Work out the finished part from the listing and answer in its coordinate system (mm). Coordinates: 2 decimals unless noted, no trailing zeros. Order: outer loops, then holes, each group sorted by start corner. A loop starts at its lowest first (then second) coordinate and runs counter-clockwise, first axis right, second up. Notation, with made-up numbers: M 4.25,31 L 54.25,31 A17 ccw 54.25,64 Z; hole C 83,-32.5 d2. An arc over 180 degrees is marked long. Write item = value, one per line. Start each with the question number.
Q1. Find section C-C on y = 0.7. Give the vertices of the cut face in (x, z) (3 decimals).
Q2. Straight lines are drawn through the part: line 1 along Z through (x, y) = (67, 0.35) (3 decimals); line 2 along X through (y, z) = (1.7, 1) (3 decimals); line 3 along Z through (x, y) = (64.5, 0.95). For each, find the intervals that lie inside material, in ascending order.
Q3. Find section A-A on z = 0. Give the vertices of the cut face in (x, y) (3 decimals).
Q4. Find section B-B on x = 70.5. Give the vertices of the cut face in (y, z) (3 decimals).
Q5. Find section D-D on x = 82.5. Give the vertices of the cut face in (y, z) (3 decimals), and give its area (3 significant figures).
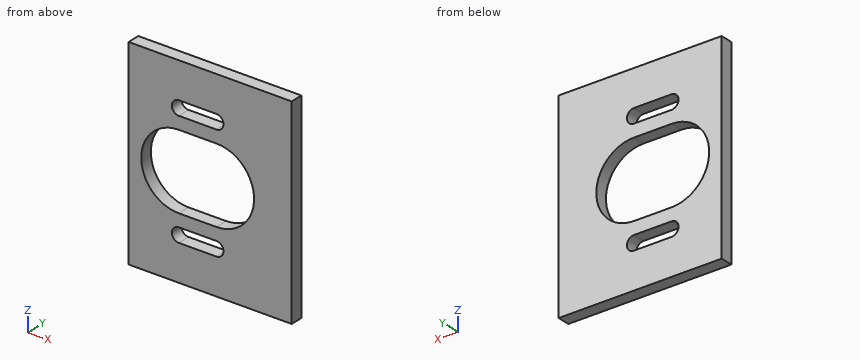
```python
from build123d import *

# Parameters (mm, degrees)
SKETCH1_W           = 177.8
SKETCH1_H           = 50.8
BOSS_EXTRUDE1_DEPTH = 3.175
CUT_EXTRUDE1_DEPTH  = 3.175
SKETCH6_W           = 142.875
SKETCH6_H           = 50.8
CUT_EXTRUDE3_DEPTH  = 3.175
SKETCH8_W           = 50.8
SKETCH8_H           = 3.175
BOSS_EXTRUDE2_DEPTH = 6.35


with BuildPart() as part:
    # Sketch1 → Boss-Extrude1 (new body)
    with BuildSketch(Plane(origin=(0, 0, 0), x_dir=(1, 0, 0), z_dir=(0, 1, 0))):
        Rectangle(SKETCH1_W, SKETCH1_H)
    extrude(amount=BOSS_EXTRUDE1_DEPTH)

    # Sketch2 → Cut-Extrude1 (cut)
    with BuildSketch(Plane(origin=(0, 3.175, 0), x_dir=(1, 0, 0), z_dir=(0, 1, 0))):
        with BuildLine():
            Line((-76.2, -12.722), (-66.675, -12.722))
            ThreePointArc((-66.675, -12.722), (-64.897, -14.5), (-66.675, -16.278))
            Line((-66.675, -16.278), (-76.2, -16.278))
            ThreePointArc((-76.2, -16.278), (-77.978, -14.5), (-76.2, -12.722))
        make_face()
        with BuildLine():
            Line((-66.675, 12.722), (-76.2, 12.722))
            ThreePointArc((-76.2, 12.722), (-77.978, 14.5), (-76.2, 16.278))
            Line((-76.2, 16.278), (-66.675, 16.278))
            ThreePointArc((-66.675, 16.278), (-64.897, 14.5), (-66.675, 12.722))
        make_face()
        with BuildLine():
            Line((-66.675, -9.525), (-76.2, -9.525))
            ThreePointArc((-76.2, -9.525), (-85.725, 0), (-76.2, 9.525))
            Line((-76.2, 9.525), (-66.675, 9.525))
            ThreePointArc((-66.675, 9.525), (-57.15, 0), (-66.675, -9.525))
        make_face()
    cut_extrude1 = extrude(amount=-CUT_EXTRUDE1_DEPTH, mode=Mode.SUBTRACT)

    # Mirror1: Cut-Extrude1 across plane
    add(cut_extrude1.mirror(Plane(origin=(0, 0, 0), x_dir=(0, 0, 1), z_dir=(1, 0, 0))), mode=Mode.SUBTRACT)

    # Sketch6 → Cut-Extrude3 (cut)
    with BuildSketch(Plane(origin=(0, 3.175, 0), x_dir=(1, 0, 0), z_dir=(0, 1, 0))):
        with Locations((-17.4625, 0)):
            Rectangle(SKETCH6_W, SKETCH6_H)
    extrude(amount=-CUT_EXTRUDE3_DEPTH, mode=Mode.SUBTRACT)

    # Sketch8 → Boss-Extrude2 (add)
    with BuildSketch(Plane(origin=(88.9, 0, 0), x_dir=(0, 0, -1), z_dir=(1, 0, 0))):
        with Locations((0, 1.5875)):
            Rectangle(SKETCH8_W, SKETCH8_H)
    extrude(amount=BOSS_EXTRUDE2_DEPTH)


solid = part.part
```
Findings below:
q1.outline = M 53.975,-25.4 L 95.25,-25.4 L 95.25,25.4 L 53.975,25.4 Z; hole M 66.675,-16.278 L 76.2,-16.278 A1.778 ccw 76.2,-12.722 L 66.675,-12.722 A1.778 ccw Z; hole M 66.675,-9.525 L 76.2,-9.525 A9.525 ccw 76.2,9.525 L 66.675,9.525 A9.525 ccw Z; hole M 66.675,12.722 L 76.2,12.722 A1.778 ccw 76.2,16.278 L 66.675,16.278 A1.778 ccw Z
q2.line_1 = -25.4 to -16.278, -12.722 to -9.525, 9.525 to 12.722, 16.278 to 25.4
q2.line_2 = 53.975 to 57.203, 85.672 to 95.25
q2.line_3 = -25.4 to -9.27, 9.27 to 25.4
q3.outline = M 53.975,0 L 57.15,0 L 57.15,3.175 L 53.975,3.175 Z; M 85.725,0 L 95.25,0 L 95.25,3.175 L 85.725,3.175 Z
q4.outline = M 0,-25.4 L 3.175,-25.4 L 3.175,-16.278 L 0,-16.278 Z; M 0,-12.722 L 3.175,-12.722 L 3.175,-9.525 L 0,-9.525 Z; M 0,9.525 L 3.175,9.525 L 3.175,12.722 L 0,12.722 Z; M 0,16.278 L 3.175,16.278 L 3.175,25.4 L 0,25.4 Z
q5.outline = M 0,-25.4 L 3.175,-25.4 L 3.175,-7.144 L 0,-7.144 Z; M 0,7.144 L 3.175,7.144 L 3.175,25.4 L 0,25.4 Z
q5.area = 116 mm^2
